The listing builds one solid part. Answer for the finished solid, in the listing's coordinates (mm). A direction names the side the tool comes from. Coordinates: 2 decimals unless noted, no trailing zeros. Loops run counter-clockwise (first coordinate to the right, second up) from the corner with the lowest first, then second, coordinate; pieces in that order, holes last. Notation, with made-up numbers: M -40,-12.75 L 5,-12.75 A11 ccw 5,4.25 Z; hole C 59.5,40.5 d11. An arc over 180 degrees is marked long. Return JSON: item names as keys, results as strings. Group by question number.
1. The mould has two halves that part along X. Classify faces 1 (the face through (0, 1, 0)), 2 (the face through (0, -12, 0)), 3 (the face through (-0.54, -5.84, -2.44)): pulls with the +X half, pulls with the -X half, needs draft (parallel to the pull), parting line crosses it, or undercut.
2. Given P1, Ø5, axis at y = 3, z = -3.5, coming from the -X side; P2, Ø4, axis at y = -4.5, z = -0.5, coming from the -X side; P3, Ø2, axis at y = -3, z = 0, coming from the +X side, each flat-ended and moving along its own axis, determine where each tip first touches the part or whether it passes through.
3. Section B-B (y = -0.75) is taken. Write down the section's boundary in (x, z), then the cut area to 3 significant figures.
4. Section D-D (z = -3.25) is taken. Write down the section's boundary in (x, y).
5. Section A-A (z = 0) is taken. Write down the section's boundary in (x, y), then the cut area to 3 significant figures.
6. Straight lines are drawn through the part: L1, parallel to Y at x = -3.25, z = 1.25; L2, parallel to Y at x = -0.25, z = 0.5; L3, parallel to Z at x = 0, y = -10.5. For each, find the intervals that lie inside material, in ascending order. Write a range as from..to.
7. Section C-C (x = -3.5) is taken. Write down the section's boundary in (y, z), then the cut area to 3 significant figures.
8. Which of the six approach directions +Z, -Z, +X, -X, +Y, -Y give full straight-line access (tool end or side, diameter ignored) to faces 4 (the face through (-0.945, 2.465, -4.256)), 5 (the face through (-0.99, 3.03, -1.74)), 6 (the face through (2, 0, -2))?
Autodesk Inventor part; units mm, degrees
ref_plane "1_XY" through (0, 0, 0) normal (0, 1, 0) x (1, 0, 0)
ref_plane "1_YZ" through (0, 0, 0) normal (1, 0, 0) x (0, 0, -1)
ref_plane "1_ZX" through (0, 0, 0) normal (0, 0, -1) x (0, 1, 0)
sketch "Sketch_1" plane through (0, 0, 0) normal (0, 0, 1) x (1, 0, 0)
  line L0 (0, -12) -> (0, 5)
  line L1 (0, 5) -> (4.36, 5)
  line L2 (4.36, 5) -> (4.36, 0)
  line L3 (4.36, 0) -> (2.5, 0)
  line L4 (2.5, 0) -> (2.5, -11.5095)
  line L5 (2.5, -11.5095) -> (2.0095, -12)
  line L6 (2.0095, -12) -> (0, -12)
  line L7 (0, -12) -> (0, 5)
revolve "Revolution1" add sketch "Sketch_1" angle 360 about axis through (0, -12, 0) along (0, -1, 0)
thread "Thread1"
sketch "Sketch_2" plane through (0, 5, 0) normal (0, 1, 0) x (1, 0, 0)
  line L0 (-2, -1.1547) -> (0, -2.3094)
  line L1 (0, -2.3094) -> (2, -1.1547)
  line L2 (2, -1.1547) -> (2, 1.1547)
  line L3 (2, 1.1547) -> (0, 2.3094)
  line L4 (0, 2.3094) -> (-2, 1.1547)
  line L5 (-2, 1.1547) -> (-2, -1.1547)
extrude "Extrusion1" cut sketch "Sketch_2" against normal blind 4
ref_plane "1_XY" through (0, 0, 0) normal (0, 1, 0) x (1, 0, 0)
ref_plane "1_YZ" through (0, 0, 0) normal (1, 0, 0) x (0, 0, -1)
ref_plane "1_ZX" through (0, 0, 0) normal (0, 0, -1) x (0, 1, 0)
ref_plane "2_XY" through (0, -12, 0) normal (0, 1, 0) x (1, 0, 0)
ref_plane "2_YZ" through (0, -12, 0) normal (1, 0, 0) x (0, 0, -1)
ref_plane "2_ZX" through (0, -12, 0) normal (0, 0, -1) x (0, 1, 0)
properties part number "11-5512_"
Worked out:
{
 "1": {"face 1": "undercut", "face 2": "needs draft", "face 3": "parting line crosses it"},
 "2": {"P1": "x = -4.24", "P2": "x = -2.5", "P3": "x = 2.5"},
 "3": {"outline": "C 0,0 d5", "area": "19.6 mm^2"},
 "4": {"outline": "M -2.91,0 L 2.91,0 L 2.91,5 L -2.91,5 Z"},
 "5": {"outline": "M -4.36,0 L -2.5,0 L -2.5,-11.51 L -2.01,-12 L 2.01,-12 L 2.5,-11.51 L 2.5,0 L 4.36,0 L 4.36,5 L 2,5 L 2,1 L -2,1 L -2,5 L -4.36,5 Z", "area": "87.4 mm^2"},
 "6": {"L1": "0..5", "L2": "-12..1", "L3": "-2.5..2.5"},
 "7": {"outline": "M 0,-2.6 L 5,-2.6 L 5,2.6 L 0,2.6 Z", "area": "26.0 mm^2"},
 "8": {"face 4": "+Y, -Y", "face 5": "+Y", "face 6": "-Y"}
}
